```python
from build123d import *

# Parameters (mm, degrees)
SKETCH1_W           = 80
SKETCH1_H           = 60
SKETCH1_R           = 2
BOSS_EXTRUDE1_DEPTH = 3
FILLET1_R           = 10


with BuildPart() as part:
    # Sketch1 → Boss-Extrude1 (new body)
    # profile 1 of 2: a face of its own
    with BuildSketch(Plane(origin=(0, 0, 0), x_dir=(1, 0, 0), z_dir=(0, 1, 0))):
        with Locations((40, 30)):
            Rectangle(SKETCH1_W, SKETCH1_H)
        with Locations(Location((40, 5, 0), (0, 0, 270))):
            Circle(SKETCH1_R, mode=Mode.SUBTRACT)
        with Locations(Location((40, 55, 0), (0, 0, 270))):
            Circle(SKETCH1_R, mode=Mode.SUBTRACT)
        with Locations(Location((5, 5, 0), (0, 0, 270))):
            Circle(SKETCH1_R, mode=Mode.SUBTRACT)
        with Locations(Location((75, 5, 0), (0, 0, 270))):
            Circle(SKETCH1_R, mode=Mode.SUBTRACT)
        with Locations(Location((75, 55, 0), (0, 0, 270))):
            Circle(SKETCH1_R, mode=Mode.SUBTRACT)
        with Locations(Location((5, 55, 0), (0, 0, 270))):
            Circle(SKETCH1_R, mode=Mode.SUBTRACT)
    # profile 2 of 2: a face of its own
    with BuildSketch(Plane(origin=(0, 0, 0), x_dir=(1, 0, 0), z_dir=(0, 1, 0))):
        Polygon((14.11809549, -96.592582629), (40, 0), (0, 0), (-25.88190451, -96.592582629), align=None)
    extrude(amount=BOSS_EXTRUDE1_DEPTH)

    # Fillet1
    fillet1_edges = [part.edges().sort_by_distance(p)[0] for p in [
        (40, 1.5, 0),
        (14.11809549, 1.5, 96.592582629),
        (-25.88190451, 1.5, 96.592582629),
        (0, 1.5, 0),
    ]]
    fillet(fillet1_edges, radius=FILLET1_R)


solid = part.part
```
Verification items for the finished model (mm, model axes). A direction names the side the tool comes from. Coordinates: 2 decimals unless noted, no trailing zeros. Order: outer loops, then holes, each group sorted by start corner. A loop starts at its lowest first (then second) coordinate and runs counter-clockwise, first axis right, second up. Notation, with made-up numbers: (-11, 48) -> (-5, 48) arc R24 cw to (-5, 69) -> close; hole circle Ø1 at (60.5, -9). An arc over 180 degrees is marked (long way). Answer as CSV lines item,"result". Start each with the question number.
1) Cross-section at D-D, the plane z = -21.5. Record the boundary of the cut face in (x, y).
2) Gauge pin test, flat ends, axial feed: pin 1 Ø3 at (x, z) = (5, -5) entering from -Y; pin 2 Ø1.5 at (x, y) = (59.5, 1.5) entering from +Z; pin 3 Ø1.5 at (y, z) = (1, -23.5) entering from -X. Record the tip position at first contact, or that the pin passes through.
3) Release check for a two-part mould opening along X. For faces 4 (the face through (77, 1, -5)), 5 (the face through (6.352, 1.479, -6.474)), 6 (the face through (12.605, 1.521, 94.47)), 7 (the face through (-11.27, 1.48, 42.06)) record: released by +X, released by -X, zero draft, split by the parting line, or undercut.
4) Cross-section at B-B, the plane z = -5. Record the boundary of the cut face in (x, y).
5) Cross-section at C-C, the plane y = 2.2. Record the boundary of the cut face in (x, z), then the cut area to 3 significant figures.
6) Set-up check for faces 1 (the face through (64, 1, 0)), 2 (the face through (0, 1, -30)), 3 (the face through (38, 1, -5)): record each of +Z, -Z, +X, -X, +Y, -Y from which the full face is reachable in a straight line by a thin tool's end or side.
7) Cross-section at A-A, the plane x = 75. Record the boundary of the cut face in (y, z), then the cut area to 3 significant figures.
8) Material ranges on L1, parallel to X at y = 1.5, z = -55; L2, parallel to Z at x = 75.5, y = 2.05; L3, parallel to Z at x = 38.5, y = 0.5, recorded low to high. Write a range as [from, to].
Conclusion:
1,outline,"(0, 0) -> (80, 0) -> (80, 3) -> (0, 3) -> close"
2,pin 1,"passes through"
2,pin 2,"stops at z = 0"
2,pin 3,"stops at x = 0"
3,face 4,"undercut"
3,face 5,"undercut"
3,face 6,"released by +X"
3,face 7,"released by -X"
4,outline,"(0, 0) -> (3, 0) -> (3, 3) -> (0, 3) -> close; (7, 0) -> (38, 0) -> (38, 3) -> (7, 3) -> close; (42, 0) -> (73, 0) -> (73, 3) -> (42, 3) -> close; (77, 0) -> (80, 0) -> (80, 3) -> (77, 3) -> close"
5,outline,"(-22.51, 84) -> (-0.34, 1.27) arc R10 cw to (0, -1.32) -> (0, -60) -> (80, -60) -> (80, 0) -> (47.67, 0) arc R10 cw to (38.01, 7.41) -> (16.1, 89.18) arc R10 ccw to (6.44, 96.59) -> (-12.85, 96.59) arc R10 ccw to start; hole circle Ø4 at (5, -55); hole circle Ø4 at (5, -5); hole circle Ø4 at (40, -55); hole circle Ø4 at (40, -5); hole circle Ø4 at (75, -55); hole circle Ø4 at (75, -5)"
5,area,"8,550 mm²"
6,face 1,"+Z, +X, +Y, -Y"
6,face 2,"-Z, -X, +Y, -Y"
6,face 3,"+Y, -Y"
7,outline,"(0, -60) -> (3, -60) -> (3, -57) -> (0, -57) -> close; (0, -53) -> (3, -53) -> (3, -7) -> (0, -7) -> close; (0, -3) -> (3, -3) -> (3, 0) -> (0, 0) -> close"
7,area,"156 mm²"
8,L1,"x = [0, 3], [7, 38], [42, 73], [77, 80]"
8,L2,"z = [-60, -56.94], [-53.06, -6.94], [-3.06, 0]"
8,L3,"z = [-60, -56.32], [-53.68, -6.32], [-3.68, 6.02]"
